```python
from build123d import *

# Parameters (mm, degrees)
SKETCH_1_R             = 5
EXTRUDE_1_DEPTH        = 37
HOLE_WIZARD_M5_1_D     = 4.2
HOLE_WIZARD_M5_1_DEPTH = 12.4
HOLE_WIZARD_M5_1_TIP   = 1.2618073
HOLE_WIZARD_M5_2_D     = 4.2
HOLE_WIZARD_M5_2_DEPTH = 12.4
HOLE_WIZARD_M5_2_TIP   = 1.2618073


with BuildPart() as part:
    # 草图1 → 凸台-拉伸1 (new body)
    with BuildSketch(Plane.XY):
        Circle(SKETCH_1_R)
    extrude(amount=EXTRUDE_1_DEPTH)

    # M5 螺纹孔1
    with Locations(Plane.XY.offset(37)):
        with Locations((0, 0)):
            Hole(HOLE_WIZARD_M5_1_D / 2, depth=HOLE_WIZARD_M5_1_DEPTH)
            with Locations((0, 0, -(HOLE_WIZARD_M5_1_DEPTH + HOLE_WIZARD_M5_1_TIP / 2))):  # 118° drill point
                Cone(0, HOLE_WIZARD_M5_1_D / 2, HOLE_WIZARD_M5_1_TIP, mode=Mode.SUBTRACT)

    # M5 螺纹孔2
    with Locations(Plane(origin=(0, 0, 0), x_dir=(-1, 0, 0), z_dir=(0, 0, -1))):
        with Locations((0, 0)):
            Hole(HOLE_WIZARD_M5_2_D / 2, depth=HOLE_WIZARD_M5_2_DEPTH)
            with Locations((0, 0, -(HOLE_WIZARD_M5_2_DEPTH + HOLE_WIZARD_M5_2_TIP / 2))):  # 118° drill point
                Cone(0, HOLE_WIZARD_M5_2_D / 2, HOLE_WIZARD_M5_2_TIP, mode=Mode.SUBTRACT)


solid = part.part
```
Here's how the part is built. I have some questions about the finished solid (model axes, mm). A direction names the side the tool comes from. Round coordinates to 2 decimals unless told otherwise and drop trailing zeros. Order: outer loops, then holes, each group sorted by start corner. A loop starts at its lowest first (then second) coordinate and runs counter-clockwise, first axis right, second up. Notation, with made-up numbers: M -35.5,-30 L 7.5,-30 A20 cw 7.5,-24 Z; hole C -36.75,33 d4. An arc over 180 degrees is marked long. Use CSV: the item, a comma, the result in double quotes.
1) I'm going to push flat-ended pins straight in: P1, Ø1.5, axis at x = -0.5, z = 26.5, coming from the -Y side; P2, Ø1, axis at y = -1, z = 24.5, coming from the +X side; P3, Ø2, axis at x = 0.5, y = 0.5, coming from the +Z side; P4, Ø4, axis at y = -3, z = 14, coming from the +X side. Where does each tip first touch, or does it pass through?
Taken from the geometry:
P1,"y = -5"
P2,"x = 4.97"
P3,"z = 24.36"
P4,"x = 4.9"
2) If we mould it in two halves opening along X, with no side actions, what happens to faces 3 (the cylindrical face through (2.003, 0.631, 6.287)), 4 (the cylindrical face through (-1.08, -4.88, 18.24)), 5 (the flat face through (1, -2.2, 0))? For each: pulls with the +X half, pulls with the -X half, needs draft (parallel to the pull), parting line crosses it, or undercut.
Taken from the geometry:
face 3,"undercut"
face 4,"parting line crosses it"
face 5,"needs draft"
3) On a 3-axis mill with a long thin cutter (end or side, diameter ignored), from which of +Z, -Z, +X, -X, +Y, -Y can I reach the whole of each face in a straight line? I mean faces 1 (the cylindrical face through (-2.003, 0.631, 30.713)), 2 (the flat face through (1, -2.2, 37)). Say none if no direction works.
Taken from the geometry:
face 1,"+Z"
face 2,"+Z, +X, -X, +Y, -Y"
4) I need wall thicknesses on line 1 along Y through (x, z) = (0, 5); line 2 along Y through (x, z) = (0.5, 35); line 3 along X through (y, z) = (-1.5, 7.5). Which ranges of each line are inside material? Lowest first, please. Write a range as [from, to].
Taken from the geometry:
line 1,"[-5, -2.1], [2.1, 5]"
line 2,"[-4.97, -2.04], [2.04, 4.97]"
line 3,"[-4.77, -1.47], [1.47, 4.77]"
5) I want a section at C-C (y = 2.75). List the corners of the cut face in (x, z) for me.
Taken from the geometry:
outline,"M -4.18,0 L 4.18,0 L 4.18,37 L -4.18,37 Z"
6) I want a section at B-B (x = 2.5). List the corners of the cut face in (y, z) for me.
Taken from the geometry:
outline,"M -4.33,0 L 4.33,0 L 4.33,37 L -4.33,37 Z"
7) I want a section at A-A (z = 30.5). List the corners of the cut face in (x, y) for me.
Taken from the geometry:
outline,"C 0,0 d10; hole C 0,0 d4.2"
